Design review of the part built by this model. Coordinates are the model's own, in mm. A direction names the side the tool comes from. Coordinates: 2 decimals unless noted, no trailing zeros. Loops run counter-clockwise (first coordinate to the right, second up) from the corner with the lowest first, then second, coordinate; pieces in that order, holes last. Notation, with made-up numbers: (-22, 67) -> (28, 67) arc R25 ccw to (28, 83) -> close; hole circle Ø3 at (47.5, 26.25). An arc over 180 degrees is marked (long way). Use a Markdown table: item, result. Add a question column.
Q1. Take a section at D-D on y = 15.25. Write out the cut boundary in (x, z), plus the area to 3 significant figures.
Q2. For probe 1 along X at (y, z) = (18.65, 0); probe 2 along Z at (x, y) = (-17.5, 18.85); probe 3 along Y at (x, z) = (8, 11), list the stretches that pass through material, from the lowest coordinate up.
Q3. For faces 5 (the face through (7.5, 9, 14)), 6 (the face through (-15.6, 18.5, 3.5)), 7 (the face through (0, 22, -6)), 8 (the face through (0, 25, -9.5)), list the 3-axis set-ups (+Z, -Z, +X, -X, +Y, -Y) from which the entire face can be reached by the end or side of a thin tool; tool diameter is ignored.
Q4. Take a section at B-B on x = 0. Write out the cut boundary in (y, z), plus the area to 3 significant figures.
Q5. Draft analysis for pull direction X (two halves, no side actions). For faces 1 (the face through (2, 20, -6)), 2 (the face through (2.385, 23.055, -8.751)), 3 (the face through (-19.1, 18.5, 1.2)), 4 (the face through (-7.5, 9, 14)), state which applies: pulls with the +X half, pulls with the -X half, needs draft (parallel to the pull), parting line crosses it, or undercut.
Q6. Clearance check with flat-ended pins moving along their axes: pin 1 Ø8 at (y, z) = (12, 2) entering from +X; pin 2 Ø1.2 at (x, y) = (0, 26.5) entering from -Z; pin 3 Ø0.5 at (x, y) = (15, 18.5) entering from -Z. State where each tip first meets the part, or that it passes through.
Q7. Take a section at A-A on z = 0. Write out the cut boundary in (x, y).
Q8. Take a section at C-C on x = -16. Write out the cut boundary in (y, z), plus the area to 3 significant figures.
from build123d import *

# Parameters (mm, degrees)
BOSS_EXTRU_1_DEPTH      = 19
ESQUISSE2_R             = 2
BOSS_EXTRU_2_DEPTH      = 1
ESQUISSE3_R             = 4.5
BOSS_EXTRU_3_DEPTH      = 1
ESQUISSE4_R             = 2.5
BOSS_EXTRU_4_DEPTH      = 8
ENL_V_MAT_EXTRU_1_DEPTH = 6


with BuildPart() as part:
    # Esquisse1 → Boss.-Extru.1 (new body)
    with BuildSketch(Plane(origin=(0, 0, 0), x_dir=(1, 0, 0), z_dir=(0, 1, 0))):
        with BuildLine():
            Line((-7.5, -11.821590418), (-7.5, -16.821590418))
            Line((-7.5, -16.821590418), (7.5, -16.821590418))
            Line((7.5, -16.821590418), (7.5, -11.821590418))
            ThreePointArc((7.5, -11.821590418), (0, 14), (-7.5, -11.821590418))
        make_face()
    extrude(amount=BOSS_EXTRU_1_DEPTH)

    # Esquisse2 → Boss.-Extru.2 (add)
    with BuildSketch(Plane(origin=(0, 19, 0), x_dir=(1, 0, 0), z_dir=(0, 1, 0))):
        with BuildLine():
            Line((13.555441712, 3.5), (17.5, 3.5))
            ThreePointArc((17.5, 3.5), (21, 0), (17.5, -3.5))
            Line((17.5, -3.5), (13.555441712, -3.5))
            ThreePointArc((13.555441712, -3.5), (14, 0), (13.555441712, 3.5))
        make_face()
        with Locations((17.5, 0)):
            Circle(ESQUISSE2_R, mode=Mode.SUBTRACT)
        with BuildLine():
            Line((-17.5, -3.5), (-13.555441712, -3.5))
            ThreePointArc((-13.555441712, -3.5), (-14, 0), (-13.555441712, 3.5))
            Line((-13.555441712, 3.5), (-17.5, 3.5))
            ThreePointArc((-17.5, 3.5), (-21, 0), (-17.5, -3.5))
        make_face()
        with Locations((-17.5, 0)):
            Circle(ESQUISSE2_R, mode=Mode.SUBTRACT)
    extrude(amount=-BOSS_EXTRU_2_DEPTH)

    # Esquisse3 → Boss.-Extru.3 (add)
    with BuildSketch(Plane(origin=(0, 19, 0), x_dir=(1, 0, 0), z_dir=(0, 1, 0))):
        with Locations((0, 8)):
            Circle(ESQUISSE3_R)
    extrude(amount=BOSS_EXTRU_3_DEPTH)

    # Esquisse4 → Boss.-Extru.4 (add)
    with BuildSketch(Plane(origin=(0, 20, 0), x_dir=(1, 0, 0), z_dir=(0, 1, 0))):
        with Locations((0, 8)):
            Circle(ESQUISSE4_R)
    extrude(amount=BOSS_EXTRU_4_DEPTH)

    # Esquisse5 → Enlèv. mat.-Extru.1 (cut)
    with BuildSketch(Plane(origin=(0, 28, 0), x_dir=(1, 0, 0), z_dir=(0, 1, 0))):
        with BuildLine():
            Line((2, 6.5), (-2, 6.5))
            ThreePointArc((-2, 6.5), (0, 5.5), (2, 6.5))
        make_face()
        with BuildLine():
            ThreePointArc((2, 9.5), (0, 10.5), (-2, 9.5))
            Line((-2, 9.5), (2, 9.5))
        make_face()
    extrude(amount=-ENL_V_MAT_EXTRU_1_DEPTH, mode=Mode.SUBTRACT)


solid = part.part
Answer list:
| question | item | result |
|---|---|---|
| 1 | outline | (-7.5, 11.82) arc R14 ccw (long way) to (7.5, 11.82) -> (7.5, 16.82) -> (-7.5, 16.82) -> close |
| 1 | area | 669 mm² |
| 2 | probe 1 | -21 to -19.5, -15.5 to 15.5, 19.5 to 21 |
| 2 | probe 2 | -3.5 to -2, 2 to 3.5 |
| 2 | probe 3 | 0 to 19 |
| 3 | face 5 | +Z, +X, +Y, -Y |
| 3 | face 6 | +Z, -X, +Y, -Y |
| 3 | face 7 | +Z, +X, -X, +Y |
| 3 | face 8 | -Z, +X, -X, +Y |
| 4 | outline | (0, -14) -> (19, -14) -> (19, -12.5) -> (20, -12.5) -> (20, -10.5) -> (22, -10.5) -> (22, -9.5) -> (28, -9.5) -> (28, -6.5) -> (22, -6.5) -> (22, -5.5) -> (20, -5.5) -> (20, -3.5) -> (19, -3.5) -> (19, 16.82) -> (0, 16.82) -> close |
| 4 | area | 623 mm² |
| 5 | face 1 | needs draft |
| 5 | face 2 | parting line crosses it |
| 5 | face 3 | undercut |
| 5 | face 4 | pulls with the -X half |
| 6 | pin 1 | x = 14 |
| 6 | pin 2 | z = -9.5 |
| 6 | pin 3 | z = -3.5 |
| 7 | outline | (-21, 18) -> (-19.5, 18) -> (-19.5, 19) -> (-21, 19) -> close; (-15.5, 18) -> (-14, 18) -> (-14, 0) -> (14, 0) -> (14, 18) -> (15.5, 18) -> (15.5, 19) -> (-15.5, 19) -> close; (19.5, 18) -> (21, 18) -> (21, 19) -> (19.5, 19) -> close |
| 8 | outline | (18, -3.5) -> (19, -3.5) -> (19, -1.32) -> (18, -1.32) -> close; (18, 1.32) -> (19, 1.32) -> (19, 3.5) -> (18, 3.5) -> close |
| 8 | area | 4.35 mm² |
